Can you work these out from the model? Positions are in its coordinate system, mm. Round coordinates to 2 decimals unless told otherwise and drop trailing zeros. Order: outer loops, then holes, each group sorted by start corner. A loop starts at its lowest first (then second) coordinate and runs counter-clockwise, first axis right, second up. Notation, with made-up numbers: (61.25, 71) - (101.25, 71) arc R24 cw to (101.25, 92) - close; hole circle Ø10 at (59.5, 82.25). An arc over 180 degrees is marked (long way). Write item = value, one per line.
Autodesk Inventor part; units mm, degrees
ref_plane "YZ Plane" through (0, 0, 0) normal (1, 0, 0) x (0, 1, 0)
ref_plane "XZ Plane" through (0, 0, 0) normal (0, 1, 0) x (-1, 0, 0)
ref_plane "XY Plane" through (0, 0, 0) normal (0, 0, 1) x (1, 0, 0)
sketch "Sketch1" plane through (0, 0, 0) normal (0, 1, 0) x (-1, 0, 0)
  line L0 (0, 0) -> (400, 0)
  line L1 (400, 0) -> (400, 300)
  line L2 (400, 300) -> (0, 300)
  line L3 (0, 300) -> (0, 0)
  dimension "d0" = 300
  dimension "d1" = 400
extrude "Extrusion1" add sketch "Sketch1" along normal blind 3.175
sketch "Sketch2" plane through (0, 3.175, 0) normal (0, 1, 0) x (1, 0, 0)
  line L0 (0, -300) -> (0, 0)
  line L1 (0, -170) -> (-25, -170)
  line L2 (-25, -170) -> (-25, -120)
  line L3 (-25, -120) -> (0, -120)
  line L4 (0, -120) -> (0, -170)
  line L5 (-400, 0) -> (-400, -300)
  line L6 (-400, -190) -> (-380, -190)
  line L7 (-380, -190) -> (-380, -140)
  line L8 (-380, -140) -> (-400, -140)
  line L9 (-400, -140) -> (-400, -190)
  line L10 (-400, -300) -> (0, -300)
  point P0 (0, -120)
  dimension "d4" = 25
  dimension "d5" = 130
  dimension "d6" = 180
  dimension "d7" = 20
  dimension "d8" = 110
  dimension "d9" = 160
extrude "Extrusion2" cut sketch "Sketch2" against normal through all
properties part number "Stock Aluminum Sheet"
(1) If I drill on line 1 (Z direction, x = -22.5, y = 2.8); line 2 (Z direction, x = -382.5, y = 0.2); line 3 (X direction, y = 2.1, z = 164), over which ranges is the centre line in solid material (lowest first)? Write a range as from..to.
Computed:
line_1 = 0..120, 170..300
line_2 = 0..140, 190..300
line_3 = -380..-25
(2) If we section it at A-A (y = 1.95): Write out the boundary of the cut face in (x, z), plus the area to 3 significant figures.
Computed:
outline = (-400, 0) - (0, 0) - (0, 120) - (-25, 120) - (-25, 170) - (0, 170) - (0, 300) - (-400, 300) - (-400, 190) - (-380, 190) - (-380, 140) - (-400, 140) - close
area = 118,000 mm^2
(3) If we section it at B-B (z = 158): Write out the boundary of the cut face in (x, y) (3 decimals).
Computed:
outline = (-380, 0) - (-25, 0) - (-25, 3.175) - (-380, 3.175) - close
(4) Will this pin go through, and if not, where does the flat tip stop? P1, Ø1.6, axis at y = 1.5, z = 174, coming from the -X side.
Computed:
P1 = -380
